```python
from build123d import *

# Parameters (mm, degrees)
F0_R     = 10
F1_DEPTH = 2
F2_R     = 1
F3_DEPTH = 3
F4_R     = 1
F5_DEPTH = 4.7


with BuildPart() as f1:
    # F0 (on Front) → F1 (new body)
    with BuildSketch(Plane.XZ):
        Circle(F0_R)
    extrude(amount=F1_DEPTH)

    # F2 (on face) → F3 (join)
    with BuildSketch(Plane.XZ.offset(2)):
        with Locations((0, 8)):
            Circle(F2_R)
        with Locations((-6.9282032303, -4)):
            Circle(F2_R)
        with Locations((6.9282032303, -4)):
            Circle(F2_R)
    extrude(amount=F3_DEPTH)

    # F4 (on face) → F5 (join)
    with BuildSketch(Plane(origin=(0, 0, 0), x_dir=(-1, 0, 0), z_dir=(0, 1, 0))):
        Circle(F4_R)
    extrude(amount=F5_DEPTH)


solid = f1.part
```
The model under review builds one solid part; all positions refer to its coordinate system, in mm. A direction names the side the tool comes from. Round coordinates to 2 decimals unless told otherwise and drop trailing zeros. Loops run counter-clockwise (first coordinate to the right, second up) from the corner with the lowest first, then second, coordinate; pieces in that order, holes last. Notation, with made-up numbers: (81, -0.75) -> (97, -0.75) arc R21 ccw to (97, 13.25) -> close; hole circle Ø3 at (42.25, 80.25). An arc over 180 degrees is marked (long way). Answer as a JSON object with one key per item and string values. Group by question number.
1) We need section D-D on z = -4. Write out the cut boundary in (x, y).
2) We need section C-C on x = 0. Write out the cut boundary in (y, z).
3) We need section B-B on y = -3.75. Write out the cut boundary in (x, z).
4) We need section A-A on z = 0. Write out the cut boundary in (x, y).
5) Mouldability with a two-part tool opening along X and no side actions: class faces 4 (the face through (7.882, -3.479, -3.7)), 5 (the face through (-7, -5, -4)), 6 (the face through (-2.17, -0.99, -9.76)) as released by +X, released by -X, zero draft, split by the parting line, or undercut.
6) For faces 1 (the face through (-7.927, -3.479, -3.956)), 2 (the face through (7, -5, -4)), 3 (the face through (0, 2, -1)), list the 3-axis set-ups (+Z, -Z, +X, -X, +Y, -Y) from which the entire face can be reached by the end or side of a thin tool; tool diameter is ignored.
7) For pin 1 Ø10 at (x, z) = (0.5, -7.5) entering from +Y; pin 2 Ø6 at (x, z) = (-2, -4.5) entering from -Y; pin 3 Ø1.5 at (y, z) = (2, 3) entering from +X; pin 4 Ø5 at (x, y) = (7, 0.5) entering from +Z, all flat-tipped, find the tip position at first contact; note any pin that passes through.
8) For line 1 (Y direction, x = -4.75, z = 0); line 2 (Z direction, x = -0.5, y = 1.5); line 3 (X direction, y = -2.25, z = -4.75), list the stretches that pass through material, from the lowest coordinate up. Write a range as [from, to].
Result set:
{
 "1": {"outline": "(-9.17, -2) -> (-7.93, -2) -> (-7.93, -5) -> (-5.93, -5) -> (-5.93, -2) -> (5.93, -2) -> (5.93, -5) -> (7.93, -5) -> (7.93, -2) -> (9.17, -2) -> (9.17, 0) -> (-9.17, 0) -> close"},
 "2": {"outline": "(-5, 7) -> (-2, 7) -> (-2, -10) -> (0, -10) -> (0, -1) -> (4.7, -1) -> (4.7, 1) -> (0, 1) -> (0, 10) -> (-2, 10) -> (-2, 9) -> (-5, 9) -> close"},
 "3": {"outline": "circle Ø2 at (-6.93, -4); circle Ø2 at (0, 8); circle Ø2 at (6.93, -4)"},
 "4": {"outline": "(-10, -2) -> (10, -2) -> (10, 0) -> (1, 0) -> (1, 4.7) -> (-1, 4.7) -> (-1, 0) -> (-10, 0) -> close"},
 "5": {"face 4": "undercut", "face 5": "zero draft", "face 6": "split by the parting line"},
 "6": {"face 1": "-Y", "face 2": "+Z, -Z, +X, -X, -Y", "face 3": "+Y"},
 "7": {"pin 1": "y = 0", "pin 2": "y = -2", "pin 3": "through", "pin 4": "z = 8.9"},
 "8": {"line 1": "[-2, 0]", "line 2": "[-0.87, 0.87]", "line 3": "[-7.59, -6.27], [6.27, 7.59]"}
}
